Source: CAD feature listing. Evaluate the final solid. Frame: model axes, mm. Face numbers are marked on the shaded views. A direction names the side the tool comes from. Give positions to 0.01 mm unless a question says otherwise; leave off trailing zeros. Order: outer loops, then holes, each group sorted by start corner. A loop starts at its lowest first (then second) coordinate and runs counter-clockwise, first axis right, second up. Notation, with made-up numbers: (84.25, 17) - (102.25, 17) arc R16 cw to (102.25, 36) - close; hole circle Ø11 at (20, 34.5). An arc over 180 degrees is marked (long way). Use CSV: the item, a comma, the result in double quotes.
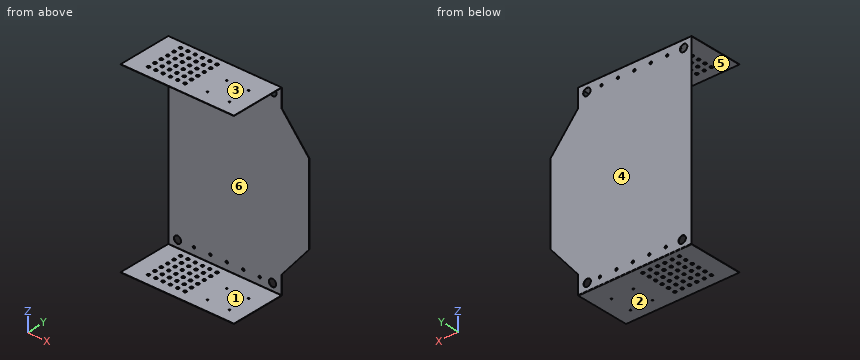
```python
from build123d import *

# Parameters (mm, degrees)
SKETCH6_R                    = 10
SKETCH6_R_2                  = 3.25
BASE_FLANGE2_DEPTH           = 1
EDGE_FLANGE1_STRIP_W         = 5.4732
EDGE_FLANGE1_STRIP_H         = 1
EDGE_FLANGE1_STRIP_CUT_DEPTH = 310
EDGE_FLANGE1_DEPTH           = 310
SKETCH23_R                   = 4
CUT_EXTRUDE1_DEPTH           = 10
SKETCH24_R                   = 2
CUT_EXTRUDE2_DEPTH           = 10


# Sheet-metal steps are written as plain solids
with BuildPart() as part:
    # Sketch6 → Base-Flange2 (new body)
    with BuildSketch(Plane(origin=(0, 0, 0), x_dir=(1, 0, 0), z_dir=(0, 1, 0))):
        Polygon((-188.372816417, 230.260729543), (-188.372816417, -269.739270457), (121.627183583, -269.739270457), (121.627183583, -219.739270457), (196.627183583, -129.739270457), (196.627183583, 90.260729543), (121.627183583, 180.260729543), (121.627183583, 230.260729543), align=None)
        with Locations(Location((-163.372816417, 210.260729543, 0), (0, 0, 270))):
            Circle(SKETCH6_R, mode=Mode.SUBTRACT)
        with Locations(Location((-118.372816417, 210.260729543, 0), (0, 0, 270))):
            Circle(SKETCH6_R_2, mode=Mode.SUBTRACT)
        with Locations(Location((-73.372816417, 210.260729543, 0), (0, 0, 270))):
            Circle(SKETCH6_R_2, mode=Mode.SUBTRACT)
        with Locations(Location((-28.372816417, 210.260729543, 0), (0, 0, 270))):
            Circle(SKETCH6_R_2, mode=Mode.SUBTRACT)
        with Locations(Location((16.627183583, 210.260729543, 0), (0, 0, 270))):
            Circle(SKETCH6_R_2, mode=Mode.SUBTRACT)
        with Locations(Location((96.627183583, 210.260729543, 0), (0, 0, 270))):
            Circle(SKETCH6_R, mode=Mode.SUBTRACT)
        with Locations(Location((61.627183583, 210.260729543, 0), (0, 0, 270))):
            Circle(SKETCH6_R_2, mode=Mode.SUBTRACT)
        with Locations(Location((-167.356668965, -249.739270457, 0), (0, 0, 90))):
            Circle(SKETCH6_R, mode=Mode.SUBTRACT)
        with Locations(Location((-122.356668965, -249.739270457, 0), (0, 0, 90))):
            Circle(SKETCH6_R_2, mode=Mode.SUBTRACT)
        with Locations(Location((-77.356668965, -249.739270457, 0), (0, 0, 90))):
            Circle(SKETCH6_R_2, mode=Mode.SUBTRACT)
        with Locations(Location((-32.356668965, -249.739270457, 0), (0, 0, 90))):
            Circle(SKETCH6_R_2, mode=Mode.SUBTRACT)
        with Locations(Location((12.643331035, -249.739270457, 0), (0, 0, 90))):
            Circle(SKETCH6_R_2, mode=Mode.SUBTRACT)
        with Locations(Location((97.643331035, -249.739270457, 0), (0, 0, 90))):
            Circle(SKETCH6_R, mode=Mode.SUBTRACT)
        with Locations(Location((57.643331035, -249.739270457, 0), (0, 0, 90))):
            Circle(SKETCH6_R_2, mode=Mode.SUBTRACT)
    extrude(amount=-BASE_FLANGE2_DEPTH)

    # Edge-Flange1 strip (across the edge) → Edge-Flange1 strip cut (cut)
    with BuildSketch(Plane(origin=(121.627183583, -1, 269.739270457), x_dir=(0, 0, -1), z_dir=(-1, 0, 0))):
        with Locations((-2, -0.5)):
            Rectangle(EDGE_FLANGE1_STRIP_W, EDGE_FLANGE1_STRIP_H)
    edge_flange1_strip_cut = extrude(amount=EDGE_FLANGE1_STRIP_CUT_DEPTH, mode=Mode.SUBTRACT)

    # Edge-Flange1 section (across the edge) → Edge-Flange1 (add)
    with BuildSketch(Plane(origin=(121.627183583, -1, 269.739270457), x_dir=(0, 0, -1), z_dir=(-1, 0, 0))):
        with BuildLine():
            Line((-1, 0.7366), (-1, 149))
            Line((-1, 149), (0, 149))
            Line((0, 149), (0, 0.7366))
            ThreePointArc((0, 0.7366), (0.215745145, 0.215745145), (0.7366, 0))
            Line((0.7366, 0), (0.7366, -1))
            ThreePointArc((0.7366, -1), (-0.491361636, -0.491361636), (-1, 0.7366))
        make_face()
    edge_flange1 = extrude(amount=EDGE_FLANGE1_DEPTH)

    # Sketch23 → Cut-Extrude1 (cut)
    with BuildSketch(Plane.XY.offset(270.739270457)):
        with Locations((-138.372816417, -120)):
            Circle(SKETCH23_R)
        with Locations((-118.372816417, -120)):
            Circle(SKETCH23_R)
        with Locations((-98.372816417, -120)):
            Circle(SKETCH23_R)
        with Locations((-78.372816417, -120)):
            Circle(SKETCH23_R)
        with Locations((-58.372816417, -120)):
            Circle(SKETCH23_R)
        with Locations((-38.372816417, -120)):
            Circle(SKETCH23_R)
        with Locations((-118.372816417, -100)):
            Circle(SKETCH23_R)
        with Locations((-98.372816417, -100)):
            Circle(SKETCH23_R)
        with Locations((-78.372816417, -100)):
            Circle(SKETCH23_R)
        with Locations((-58.372816417, -100)):
            Circle(SKETCH23_R)
        with Locations((-38.372816417, -100)):
            Circle(SKETCH23_R)
        with Locations((-118.372816417, -80)):
            Circle(SKETCH23_R)
        with Locations((-98.372816417, -80)):
            Circle(SKETCH23_R)
        with Locations((-78.372816417, -80)):
            Circle(SKETCH23_R)
        with Locations((-58.372816417, -80)):
            Circle(SKETCH23_R)
        with Locations((-38.372816417, -80)):
            Circle(SKETCH23_R)
        with Locations((-118.372816417, -60)):
            Circle(SKETCH23_R)
        with Locations((-98.372816417, -60)):
            Circle(SKETCH23_R)
        with Locations((-78.372816417, -60)):
            Circle(SKETCH23_R)
        with Locations((-58.372816417, -60)):
            Circle(SKETCH23_R)
        with Locations((-38.372816417, -60)):
            Circle(SKETCH23_R)
        with Locations((-118.372816417, -40)):
            Circle(SKETCH23_R)
        with Locations((-98.372816417, -40)):
            Circle(SKETCH23_R)
        with Locations((-78.372816417, -40)):
            Circle(SKETCH23_R)
        with Locations((-58.372816417, -40)):
            Circle(SKETCH23_R)
        with Locations((-38.372816417, -40)):
            Circle(SKETCH23_R)
        with Locations((-118.372816417, -20)):
            Circle(SKETCH23_R)
        with Locations((-98.372816417, -20)):
            Circle(SKETCH23_R)
        with Locations((-78.372816417, -20)):
            Circle(SKETCH23_R)
        with Locations((-58.372816417, -20)):
            Circle(SKETCH23_R)
        with Locations((-38.372816417, -20)):
            Circle(SKETCH23_R)
        with Locations((-138.372816417, -100)):
            Circle(SKETCH23_R)
        with Locations((-138.372816417, -80)):
            Circle(SKETCH23_R)
        with Locations((-138.372816417, -60)):
            Circle(SKETCH23_R)
        with Locations((-138.372816417, -40)):
            Circle(SKETCH23_R)
        with Locations((-138.372816417, -20)):
            Circle(SKETCH23_R)
    cut_extrude1 = extrude(amount=-CUT_EXTRUDE1_DEPTH, mode=Mode.SUBTRACT)

    # Sketch24 → Cut-Extrude2 (cut)
    with BuildSketch(Plane.XY.offset(270.739270457)):
        with Locations((18.484920525, -55)):
            Circle(SKETCH24_R)
        with Locations(Location((78.484920525, -55, 0), (0, 0, 90))):
            Circle(SKETCH24_R)
        with Locations((78.484920525, -115)):
            Circle(SKETCH24_R)
        with Locations(Location((18.484920525, -115, 0), (0, 0, 90))):
            Circle(SKETCH24_R)
    cut_extrude2 = extrude(amount=-CUT_EXTRUDE2_DEPTH, mode=Mode.SUBTRACT)

    # Mirror2: Edge-Flange1 strip cut, Edge-Flange1, Cut-Extrude1 across plane
    add(edge_flange1_strip_cut.mirror(Plane(origin=(0, 0, 19.739270457), x_dir=(1, 0, 0), z_dir=(0, 0, -1))), mode=Mode.SUBTRACT)
    add(edge_flange1.mirror(Plane(origin=(0, 0, 19.739270457), x_dir=(1, 0, 0), z_dir=(0, 0, -1))))
    add(cut_extrude1.mirror(Plane(origin=(0, 0, 19.739270457), x_dir=(1, 0, 0), z_dir=(0, 0, -1))), mode=Mode.SUBTRACT)

    # Mirror3: Cut-Extrude2 across plane
    add(cut_extrude2.mirror(Plane(origin=(0, 0, 19.739270457), x_dir=(1, 0, 0), z_dir=(0, 0, -1))), mode=Mode.SUBTRACT)


solid = part.part
```
Item 1: Material intervals for line 1 (Z direction, x = 80.5, y = -25); line 2 (Y direction, x = 64.5, z = 61.5), sorted ascending. Write a range as from..to.
Filled in:
line 1,"z = -231.26..-230.26, 269.74..270.74"
line 2,"y = -1..0"
Item 2: First-contact query: pin 1 (1 mm diameter, centred on x = -141.5, z = -168, fed in from -Y). Flat tip, straight axial feed; report the tip coordinate or a pass-through.
Filled in:
pin 1,"stops at y = -1"
Item 3: Section B-B on z = -114. Return the cut outline in (x, y), then the cut area to 3 significant figures.
Filled in:
outline,"(-188.37, -1) - (176.84, -1) - (176.84, 0) - (-188.37, 0) - close"
area,"365 mm2"
Item 4: Section C-C on z = 98.5. Return the cut outline in (x, y), then the cut area to 3 significant figures.
Filled in:
outline,"(-188.37, -1) - (196.63, -1) - (196.63, 0) - (-188.37, 0) - close"
area,"385 mm2"
Item 5: Section A-A on x = -89. Return the cut outline in (y, z), then the cut area to 3 significant figures.
Filled in:
outline,"(-150, -231.26) - (-1.74, -231.26) arc R1.74 ccw to (0, -229.52) - (0, 269) arc R1.74 ccw to (-1.74, 270.74) - (-150, 270.74) - (-150, 269.74) - (-1.74, 269.74) arc R0.74 cw to (-1, 269) - (-1, -229.52) arc R0.74 cw to (-1.74, -230.26) - (-150, -230.26) - close"
area,"799 mm2"
Item 6: Mould query, pull axis Z, two halves, no side actions, for the marked faces 3, 4, 5 and 6. Classes: released by +Z, released by -Z, zero draft, split by the parting line, or undercut.
Filled in:
face 3,"released by +Z"
face 4,"zero draft"
face 5,"undercut"
face 6,"undercut"
Item 7: Set-up query: the marked faces 1 and 2. Return all of +Z, -Z, +X, -X, +Y, -Y with unobstructed straight access to the full face (end or side cutting, diameter ignored); none if empty.
Filled in:
face 1,"+X, -X, -Y"
face 2,"-Z, +X, -X, +Y, -Y"
